Build history of the part. All positions in model axes, mm. Face numbers are marked on the shaded views. A direction names the side the tool comes from. Give positions to 0.01 mm unless a question says otherwise; leave off trailing zeros. Loops run counter-clockwise (first coordinate to the right, second up) from the corner with the lowest first, then second, coordinate; pieces in that order, holes last. Notation, with made-up numbers: (81, 49) -> (140, 49) arc R33 ccw to (140, 84) -> close; hole circle Ø5 at (-5.75, 24). An arc over 180 degrees is marked (long way). Answer as a JSON object with one key per item and string values. Group by question number.
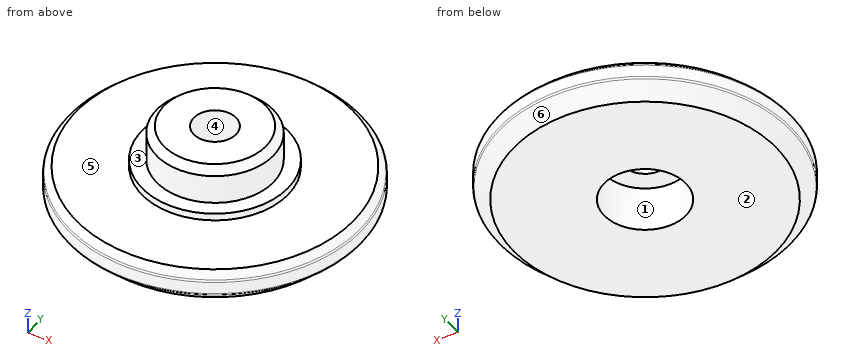
from build123d import *

# Parameters (mm, degrees)
F0_R      = 4
F1_DEPTH  = 5.5
F2_R      = 5
F3_DEPTH  = 3
F4_R      = 10
F5_DEPTH  = 2.5
F6_SIZE   = 1
F7_SIZE   = 0.5
F8_R      = 0.2
F9_SIZE   = 0.5
F11_R     = 2.8
F12_DEPTH = 3.1
F13_R     = 1.45
F14_DEPTH = 8.4


with BuildPart() as f1:
    # F0 (on Top) → F1 (new body)
    with BuildSketch(Plane.XY):
        Circle(F0_R)
    extrude(amount=F1_DEPTH)

    # F2 (on Top) → F3 (join)
    with BuildSketch(Plane.XY):
        Circle(F2_R)
    extrude(amount=F3_DEPTH)

    # F4 (on Top) → F5 (join)
    with BuildSketch(Plane.XY):
        Circle(F4_R)
    extrude(amount=F5_DEPTH)

    # F6
    f6_edges = [f1.edges().sort_by_distance(p)[0] for p in [
        (-10, 0, 0),
    ]]
    chamfer(f6_edges, length=F6_SIZE)

    # F7
    f7_edges = [f1.edges().sort_by_distance(p)[0] for p in [
        (-10, 0, 2.5),
    ]]
    chamfer(f7_edges, length=F7_SIZE)

    # F8
    f8_edges = [f1.edges().sort_by_distance(p)[0] for p in [
        (-10, 0, 1),
        (-10, 0, 2),
    ]]
    fillet(f8_edges, radius=F8_R)

    # F9
    f9_edges = [f1.edges().sort_by_distance(p)[0] for p in [
        (-4, 0, 5.5),
    ]]
    chamfer(f9_edges, length=F9_SIZE)


with BuildPart() as f10_1:
    # F10: copy of F1
    add(f1.part.moved(Location((-25, 0, 0))))


with BuildPart() as f1_1:
    add(f1.part)

    # F11 (on Top) → F12 (cut)
    with BuildSketch(Plane.XY):
        Circle(F11_R)
    extrude(amount=F12_DEPTH, mode=Mode.SUBTRACT)

    # F13 (on Top) → F14 (cut)
    with BuildSketch(Plane.XY):
        Circle(F13_R)
    extrude(amount=F14_DEPTH, mode=Mode.SUBTRACT)


with BuildPart() as f16_1:
    # F16: copy of F1
    add(f1_1.part.moved(Location((-23.4, 0, 0))))


solid = f1_1.part
(1) Probe line 1 along X through (y, z) = (0, 4.25); line 2 along Y through (x, z) = (0, 1.35); line 3 along Z through (x, y) = (-7, -5.5). List the from-to ranges inside material, lowest first. Write a range as [from, to].
(2) Pull direction X, two halves, no side cores. Call the marked faces 4, 5 and 6: pulls with the +X half, pulls with the -X half, needs draft (parallel to the pull), parting line crosses it, or undercut.
(3) Saw through at A-A on z = 4.65. List the corners of the cut face in (x, y), plus the area to 3 significant figures.
(4) 3-axis set-ups, long thin cutter, end or side, ignore diameter. For the marked faces 1, 2 and 3: which of +Z, -Z, +X, -X, +Y, -Y reach the whole face in a straight line?
(5) Pin check, flat tips, straight feed: pin 1 (1.7 mm diameter, centred on x = -0.5, y = 0.5, fed in from -Z); pin 2 (3 mm diameter, centred on x = 7, z = 1, fed in from +Y); pin 3 (3 mm diameter, centred on y = 3, z = 2, fed in from +X). Stop position of each tip, or through.
Calculated:
{
 "1": {"line 1": "x = [-4, -1.45], [1.45, 4]", "line 2": "y = [-10, -2.8], [2.8, 10]", "line 3": "z = [0, 2.5]"},
 "2": {"face 4": "undercut", "face 5": "needs draft", "face 6": "parting line crosses it"},
 "3": {"outline": "circle Ø8 at (0, 0); hole circle Ø2.9 at (0, 0)", "area": "43.7 mm^2"},
 "4": {"face 1": "-Z", "face 2": "-Z, +X, -X, +Y, -Y", "face 3": "+Z"},
 "5": {"pin 1": "stops at z = 3.1", "pin 2": "stops at y = 8.35", "pin 3": "stops at x = 9.89"}
}
